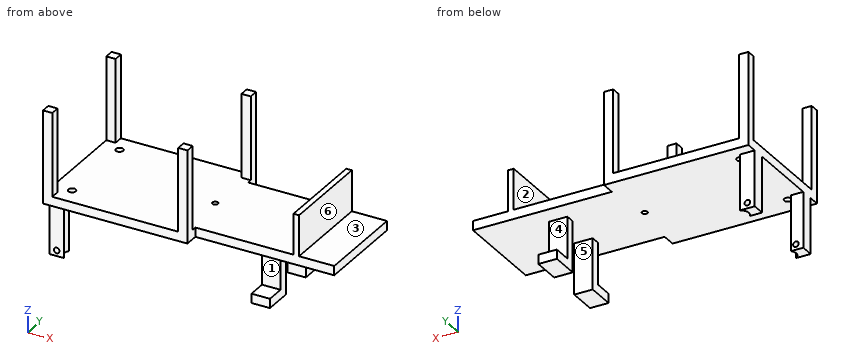
from build123d import *

# Parameters (mm, degrees)
CROQUIS1_R               = 2
CROQUIS1_R_2             = 1.5
CROQUIS1_W               = 75
CROQUIS1_H               = 50
SALIENTE_EXTRUIR4_DEPTH  = 5
CROQUIS3_W               = 5
CROQUIS3_H               = 5
SALIENTE_EXTRUIR5_DEPTH  = 50
CROQUIS4_W               = 3
CROQUIS4_H               = 50
SALIENTE_EXTRUIR7_DEPTH  = 22
SALIENTE_EXTRUIR9_DEPTH  = 27.5
CROQUIS7_W               = 10
CROQUIS7_H               = 5
SALIENTE_EXTRUIR10_DEPTH = 10
CROQUIS8_W               = 10
CROQUIS8_H               = 5
SALIENTE_EXTRUIR11_DEPTH = 10
SALIENTE_EXTRUIR12_DEPTH = 30
CROQUIS10_R              = 1.5
CORTAR_EXTRUIR1_DEPTH    = 77


with BuildPart() as part:
    # Croquis1 → Saliente-Extruir4 (new body)
    # profile 1 of 2: a face of its own
    with BuildSketch(Plane.XY):
        Polygon((-71.5, -27.5), (-71.5, -32.5), (-3.5, -32.5), (-3.5, -27.5), (1.5, -27.5), (1.5, -25), (1.5, 25), (1.5, 27.5), (-3.5, 27.5), (-3.5, 32.5), (-71.5, 32.5), (-71.5, 27.5), (-76.5, 27.5), (-76.5, -27.5), align=None)
        with Locations((-66.5, -22.5)):
            Circle(CROQUIS1_R, mode=Mode.SUBTRACT)
        with Locations((-2, 0)):
            Circle(CROQUIS1_R_2, mode=Mode.SUBTRACT)
        with Locations((-66.5, 22.5)):
            Circle(CROQUIS1_R, mode=Mode.SUBTRACT)
    # profile 2 of 2: a face of its own
    with BuildSketch(Plane.XY):
        with Locations((39, 0)):
            Rectangle(CROQUIS1_W, CROQUIS1_H)
    extrude(amount=SALIENTE_EXTRUIR4_DEPTH)

    # Croquis3 → Saliente-Extruir5 (add)
    with BuildSketch(Plane(origin=(0, 0, 0), x_dir=(-1, 0, 0), z_dir=(0, 0, -1))):
        with Locations((74, 30)):
            Rectangle(CROQUIS3_W, CROQUIS3_H)
        with Locations((1, -30)):
            Rectangle(CROQUIS3_W, CROQUIS3_H)
        with Locations((1, 30)):
            Rectangle(CROQUIS3_W, CROQUIS3_H)
        with Locations((74, -30)):
            Rectangle(CROQUIS3_W, CROQUIS3_H)
    extrude(amount=-SALIENTE_EXTRUIR5_DEPTH)

    # Croquis4 → Saliente-Extruir7 (add)
    with BuildSketch(Plane.XY.offset(5)):
        with Locations((56, 0)):
            Rectangle(CROQUIS4_W, CROQUIS4_H)
    extrude(amount=SALIENTE_EXTRUIR7_DEPTH)

    # Croquis6 → Saliente-Extruir9 (add)
    with BuildSketch(Plane(origin=(0, 0, 0), x_dir=(-1, 0, 0), z_dir=(0, 0, -1))):
        Polygon((-31.5, 13.5), (-31.5, 14.5), (-41.5, 14.5), (-41.5, 13.5), (-41.5, 9.5), (-31.5, 9.5), align=None)
        Polygon((-31.5, -13.5), (-31.5, -9.5), (-41.5, -9.5), (-41.5, -13.5), (-41.5, -14.5), (-31.5, -14.5), align=None)
    extrude(amount=SALIENTE_EXTRUIR9_DEPTH)

    # Croquis7 → Saliente-Extruir10 (add)
    with BuildSketch(Plane(origin=(0, 14.5, 0), x_dir=(1, 0, 0), z_dir=(0, 1, 0))):
        with Locations((36.5, 25)):
            Rectangle(CROQUIS7_W, CROQUIS7_H)
    extrude(amount=SALIENTE_EXTRUIR10_DEPTH)

    # Croquis8 → Saliente-Extruir11 (add)
    with BuildSketch(Plane.XZ.offset(14.5)):
        with Locations((36.5, -25)):
            Rectangle(CROQUIS8_W, CROQUIS8_H)
    extrude(amount=SALIENTE_EXTRUIR11_DEPTH)

    # Croquis9 → Saliente-Extruir12 (add)
    with BuildSketch(Plane(origin=(0, 0, 0), x_dir=(-1, 0, 0), z_dir=(0, 0, -1))):
        with BuildLine():
            Line((69.854101966, -19.5), (76.5, -19.5))
            Line((76.5, -19.5), (76.5, -26.5))
            Line((76.5, -26.5), (68.561552813, -26.5))
            ThreePointArc((68.561552813, -26.5), (70.925192558, -23.317111271), (69.854101966, -19.5))
        make_face()
        with BuildLine():
            Line((68.561552813, 26.5), (76.5, 26.5))
            Line((76.5, 26.5), (76.5, 19.5))
            Line((76.5, 19.5), (69.854101966, 19.5))
            ThreePointArc((69.854101966, 19.5), (70.925192558, 23.317111271), (68.561552813, 26.5))
        make_face()
    extrude(amount=SALIENTE_EXTRUIR12_DEPTH)

    # Croquis10 → Cortar-Extruir1 (cut)
    with BuildSketch(Plane(origin=(0, 26.5, 0), x_dir=(1, 0, 0), z_dir=(0, 1, 0))):
        with Locations(Location((-72.530776406, 27, 0), (0, 0, 270))):
            Circle(CROQUIS10_R)
    extrude(amount=-CORTAR_EXTRUIR1_DEPTH, mode=Mode.SUBTRACT)


solid = part.part
Verification items for the finished model (mm, model axes). Face numbers are marked on the shaded views. A direction names the side the tool comes from. Round coordinates to 2 decimals unless told otherwise and drop trailing zeros. Loops run counter-clockwise (first coordinate to the right, second up) from the corner with the lowest first, then second, coordinate; pieces in that order, holes last. Notation, with made-up numbers: M 79,11 L 125,11 A21 cw 125,27 Z; hole C 12,23.25 d9. An arc over 180 degrees is marked long. Write each question's results on one line, items separated by ' | '.
1) Section check C-C on y = 22.5. Record the boundary of the cut face in (x, z).
Checks:
outline: M -76.5,-30 L -71,-30 L -71,0 L -68.5,0 L -68.5,5 L -76.5,5 Z; M -64.5,0 L 76.5,0 L 76.5,5 L 57.5,5 L 57.5,27 L 54.5,27 L 54.5,5 L -64.5,5 Z; M 31.5,-27.5 L 41.5,-27.5 L 41.5,-22.5 L 31.5,-22.5 Z; hole C -72.53,-27 d3
2) Mould release check, pull along Z, two halves, no side actions. Record for the marked faces 1, 2, 3 and 4: released by +Z, released by -Z, zero draft, split by the parting line, or undercut.
Checks:
face 1: undercut | face 2: zero draft | face 3: released by +Z | face 4: undercut
3) Section check B-B on z = 10. Record the boundary of the cut face in (x, y).
Checks:
outline: M -76.5,-32.5 L -71.5,-32.5 L -71.5,-27.5 L -76.5,-27.5 Z; M -76.5,27.5 L -71.5,27.5 L -71.5,32.5 L -76.5,32.5 Z; M -3.5,-32.5 L 1.5,-32.5 L 1.5,-27.5 L -3.5,-27.5 Z; M -3.5,27.5 L 1.5,27.5 L 1.5,32.5 L -3.5,32.5 Z; M 54.5,-25 L 57.5,-25 L 57.5,25 L 54.5,25 Z
4) Section check D-D on x = -66.5. Record the boundary of the cut face in (y, z), then the cut area to 3 significant figures.
Checks:
outline: M -32.5,0 L -24.5,0 L -24.5,5 L -32.5,5 Z; M -20.5,0 L 20.5,0 L 20.5,5 L -20.5,5 Z; M 24.5,0 L 32.5,0 L 32.5,5 L 24.5,5 Z | area: 285 mm2
5) Section check A-A on z = -18.5. Record the boundary of the cut face in (x, y), then the cut area to 3 significant figures.
Checks:
outline: M -76.5,-26.5 L -68.56,-26.5 A4.5 cw -69.85,-19.5 L -76.5,-19.5 Z; M -76.5,19.5 L -69.85,19.5 A4.5 cw -68.56,26.5 L -76.5,26.5 Z; M 31.5,-14.5 L 41.5,-14.5 L 41.5,-9.5 L 31.5,-9.5 Z; M 31.5,9.5 L 41.5,9.5 L 41.5,14.5 L 31.5,14.5 Z | area: 185 mm2
6) Access from +Z, -Z, +X, -X, +Y, -Y to the whole of each face (thin tool, end or side, straight path). Record for the marked faces 5 and 6.
Checks:
face 5: -Z, +X, -X | face 6: +Z, +X, +Y, -Y
7) Scan lines: L1, parallel to Y at x = -66.5, z = 3.75; L2, parallel to Y at x = -2, z = 4; L3, parallel to Z at x = 36, y = 17. Record each from-to range of solid material in increasing order. Write a range as from..to.
Checks:
L1: y = -32.5..-24.5, -20.5..20.5, 24.5..32.5 | L2: y = -32.5..-1.5, 1.5..32.5 | L3: z = -27.5..-22.5, 0..5
8) Gauge pin test, flat ends, axial feed: P1, Ø3.5, axis at x = 55.5, y = -5.5, coming from the +Z side; P2, Ø6, axis at x = 12.5, y = 6, coming from the -Z side; P3, Ø2, axis at x = 48.5, y = 20, coming from the +Z side. Record the tip position at first contact, or that the pin passes through.
Checks:
P1: stops at z = 27 | P2: stops at z = 0 | P3: stops at z = 5
